Autodesk Inventor part; units mm, degrees
ref_plane "YZ Plane" through (0, 0, 0) normal (1, 0, 0) x (0, 1, 0)
ref_plane "XZ Plane" through (0, 0, 0) normal (0, 1, 0) x (-1, 0, 0)
ref_plane "XY Plane" through (0, 0, 0) normal (0, 0, 1) x (1, 0, 0)
sketch "Sketch2" plane through (0, 0, 0) normal (0, 0, 1) x (1, 0, 0)
  line L0 (99.5, 55) -> (-99.5, 55)
  line L1 (-99.5, 55) -> (-99.5, -55)
  line L2 (-99.5, -55) -> (99.5, -55)
  line L3 (99.5, -55) -> (99.5, 55)
  line L4 (99.5, 55) -> (-99.5, -55) construction
  line L5 (-99.5, 55) -> (99.5, -55) construction
  point P0 (0, 0)
  dimension "d4" = 199
  dimension "d5" = 110
extrude "Extrusion2" add sketch "Sketch2" along normal blind 2
sketch "Sketch3" plane through (0, 0, 2) normal (0, 0, 1) x (1, 0, 0)
  line L0 (99.5, -55) -> (99.5, 55)
  line L1 (-99.5, 55) -> (99.5, 55)
  line L2 (99.5, 55) -> (99.5, 53)
  line L3 (99.5, 53) -> (-99.5, 53)
  line L4 (-99.5, 53) -> (-99.5, 55)
  point P0 (0, 0)
  dimension "d8" = 2
extrude "Extrusion3" add sketch "Sketch3" along normal blind 48
fillet "Fillet1" radius 1 2 edges at (0, 55, 0) (0, 53, 2)
properties part number "supply base"
Model file for the job. Use its own axes, mm. A direction names the side the tool comes from. Coordinates: 2 decimals unless noted, no trailing zeros. Order: outer loops, then holes, each group sorted by start corner. A loop starts at its lowest first (then second) coordinate and runs counter-clockwise, first axis right, second up. Notation, with made-up numbers: M 30.25,47.5 L 54.25,47.5 A14 ccw 54.25,64.5 Z; hole C -10.5,36.25 d10. An arc over 180 degrees is marked long. Answer as CSV lines item,"result".
(1) Band-saw the part on A-A, the plane x = 59. List the corners of the cut face in (y, z).
Geometry says:
outline,"M -55,0 L 54,0 A1 ccw 55,1 L 55,50 L 53,50 L 53,3 A1 cw 52,2 L -55,2 Z"
(2) Wall check: line 1 along Z through (x, y) = (-67, -20); line 2 along Y through (x, z) = (-15, 42.5). Give the ranges that are in metal, low to high.
Geometry says:
line 1,"z = 0 to 2"
line 2,"y = 53 to 55"
(3) 3-axis set-ups, long thin cutter, end or side, ignore diameter. For faces 1 (the flat face through (-1, 0, 0)), 2 (the flat face through (1, 53, 26)): which of +Z, -Z, +X, -X, +Y, -Y reach the whole face in a straight line?
Geometry says:
face 1,"-Z, +X, -X, +Y, -Y"
face 2,"+Z, +X, -X, -Y"
(4) Flat gauge pins, fed straight in: pin 1 (3 mm diameter, centred on x = 51, y = 3.5, fed in from +Z); pin 2 (14 mm diameter, centred on x = -22, z = 21, fed in from -Y); pin 3 (12 mm diameter, centred on y = -6.5, z = 9.5, fed in from -X); pin 4 (5 mm diameter, centred on x = 72, y = 26, fed in from -Z). Where does each tip first touch, or does it go through?
Geometry says:
pin 1,"stops at z = 2"
pin 2,"stops at y = 53"
pin 3,"passes through"
pin 4,"stops at z = 0"
(5) Band-saw the part on C-C, the plane y = -43. List the corners of the cut face in (x, z).
Geometry says:
outline,"M -99.5,0 L 99.5,0 L 99.5,2 L -99.5,2 Z"
(6) Band-saw the part on B-B, the plane z = 46.5. List the corners of the cut face in (x, y), then the cut area to 3 significant figures.
Geometry says:
outline,"M -99.5,53 L 99.5,53 L 99.5,55 L -99.5,55 Z"
area,"398 mm2"
